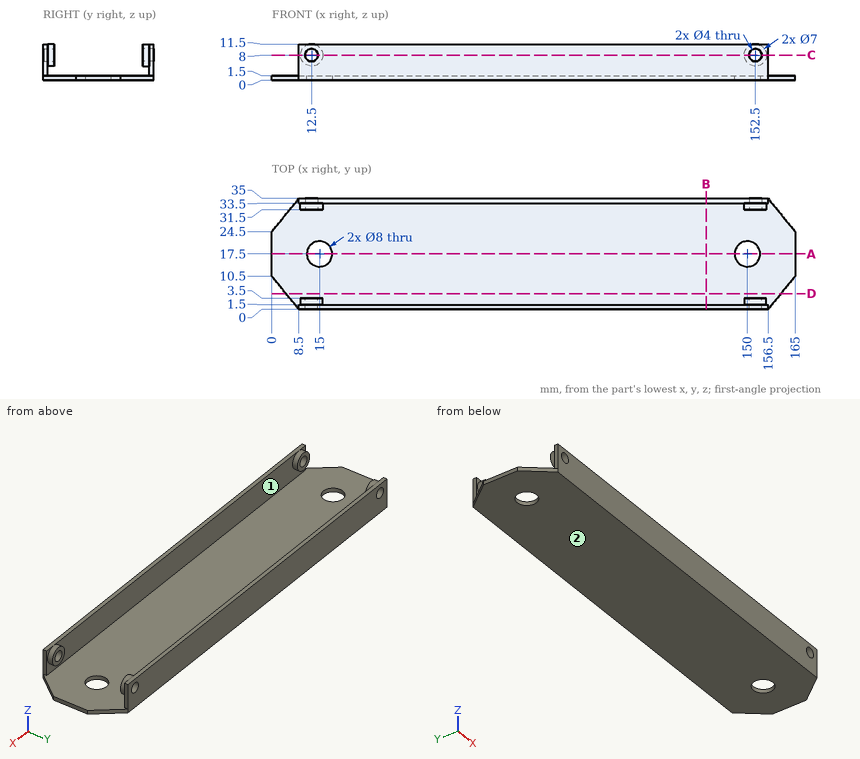
Answer from the drawing. Dimensions are ordinates in mm from the lowest x, y and z of the part. Round coordinates to 2 decimals unless told otherwise and drop trailing zeros. Order: outer loops, then holes, each group sorted by start corner. A loop starts at its lowest first (then second) coordinate and runs counter-clockwise, first axis right, second up.
1) Flat-ended cylindrical pins translate along their axes: pin 1 (3.5 mm diameter, centred on x = 152.5, z = 8, fed in from -Y); pin 2 (13 mm diameter, centred on x = 15, y = 17.5, fed in from +Z); pin 3 (0.5 mm diameter, centred on y = 1, z = 5, fed in from -X); pin 4 (0.8 mm diameter, centred on y = 34.5, z = 6.5, fed in from +X). Find the tip coordinate at first contact, or state that the pin passes through.
2) Straight lines are drawn through the part: L1, parallel to Z at x = 152.5, y = 32.35; L2, parallel to Y at x = 59.5, z = 10.5; L3, parallel to Y at x = 15, z = 0.6. For each, find the intervals that lie inside material, in ascending order.
3) The part is cut by section C-C on z = 8. Give the number of separate pieces and of enclosed holes in the cut face, plus the area to 3 significant figures.
4) The part is cut by section B-B on x = 137. Write down the section's boundary in (y, z).
5) The part is cut by section A-A on y = 17.5. Write down the section's boundary in (x, z), plus the area to 4 significant figures.
6) The mould has two halves that part along X. Classify the marked faces 1 and 2: released by +X, released by -X, zero draft, split by the parting line, or undercut.
7) The part is cut by section D-D on y = 5. Write down the section's boundary in (x, z).
Resolved:
1. pin 1: passes through
1. pin 2: stops at z = 1.5
1. pin 3: stops at x = 8.5
1. pin 4: stops at x = 156.5
2. L1: z = 0 to 1.5, 4.5 to 6, 10 to 11.5
2. L2: y = 0 to 1.5, 33.5 to 35
2. L3: y = 0 to 13.5, 21.5 to 35
3. separate pieces: 6
3. enclosed holes: 0
3. area: 444 mm2
4. outline: (0, 0) - (35, 0) - (35, 11.5) - (33.5, 11.5) - (33.5, 1.5) - (1.5, 1.5) - (1.5, 11.5) - (0, 11.5) - close
5. outline: (0, 0) - (11, 0) - (11, 1.5) - (0, 1.5) - close; (19, 0) - (146, 0) - (146, 1.5) - (19, 1.5) - close; (154, 0) - (165, 0) - (165, 1.5) - (154, 1.5) - close
5. area: 223.5 mm2
6. face 1: undercut
6. face 2: zero draft
7. outline: (4.45, 0) - (160.55, 0) - (160.55, 1.5) - (4.45, 1.5) - close
